from build123d import *

# Parameters (mm, degrees)
SKETCH_1_W      = 8.2
SKETCH_1_H      = 5.2
EXTRUDE_1_DEPTH = 13
SKETCH_2_R      = 2.5
EXTRUDE_2_DEPTH = 6
SKETCH_3_R      = 1.25
EXTRUDE_3_DEPTH = 9.5


with BuildPart() as part:
    # 草圖1 → 填料-伸長1 (new body)
    with BuildSketch(Plane.XY):
        with Locations((-38.465519845, -46.707444045)):
            Rectangle(SKETCH_1_W, SKETCH_1_H)
    extrude(amount=EXTRUDE_1_DEPTH)

    # 草圖2 → 填料-伸長2 (add)
    with BuildSketch(Plane(origin=(0, 0, 0), x_dir=(-1, 0, 0), z_dir=(0, 0, -1))):
        with Locations((38.465519845, -46.707444045)):
            Circle(SKETCH_2_R)
    extrude(amount=EXTRUDE_2_DEPTH)

    # 草圖3 → 填料-伸長3 (add)
    with BuildSketch(Plane(origin=(0, 0, -6), x_dir=(-1, 0, 0), z_dir=(0, 0, -1))):
        with Locations((38.465519845, -46.707444045)):
            Circle(SKETCH_3_R)
    extrude(amount=EXTRUDE_3_DEPTH)


solid = part.part
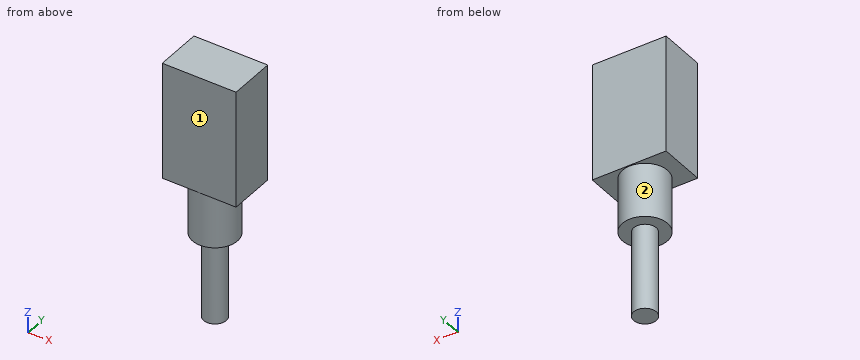
The listing builds one solid part. Answer for the finished solid, in the listing's coordinates (mm). Face numbers are marked on the shaded views. A direction names the side the tool comes from. Round coordinates to 2 decimals unless told otherwise and drop trailing zeros. Order: outer loops, then holes, each group sorted by start corner. A loop starts at its lowest first (then second) coordinate and runs counter-clockwise, first axis right, second up. Notation, with made-up numbers: M -37.5,-5.75 L -16.5,-5.75 A30 ccw -16.5,20.25 Z; hole C 32.5,72.5 d2. An arc over 180 degrees is marked long. Answer in a Markdown table with one row per item. Add a question column.
1) The part is cut by section D-D on x = -39.25. Determine the outline of the cut face in (y, z).
2) The part is cut by section C-C on y = -48.55. Determine the outline of the cut face in (x, z), plus the area to 3 significant figures.
3) Consider line 1 along Z through (x, y) = (-35.5, -48.9); line 2 along Z through (x, y) = (-38.5, -44.8); line 3 along Y through (x, z) = (-40, -3.5). Determine where each line is inside the solid, lowest interval first. Write a range as from..to.
4) Which of the six approach directions +Z, -Z, +X, -X, +Y, -Y give full straight-line access (tool end or side, diameter ignored) to the marked faces 1 and 2?
5) The part is cut by section B-B on y = -45.2. Determine the outline of the cut face in (x, z).
6) The part is cut by section A-A on x = -37.75. Determine the outline of the cut face in (y, z).
Findings below:
| question | item | result |
|---|---|---|
| 1 | outline | M -49.31,0 L -49.08,0 L -49.08,-6 L -47.68,-6 L -47.68,-15.5 L -45.73,-15.5 L -45.73,-6 L -44.33,-6 L -44.33,0 L -44.11,0 L -44.11,13 L -49.31,13 Z |
| 2 | outline | M -42.57,0 L -40.16,0 L -40.16,-6 L -36.78,-6 L -36.78,0 L -34.37,0 L -34.37,13 L -42.57,13 Z |
| 2 | area | 127 mm² |
| 3 | line 1 | z = 0..13 |
| 3 | line 2 | z = -6..13 |
| 3 | line 3 | y = -48.68..-44.73 |
| 4 | face 1 | +Z, -Z, +X, -X, -Y |
| 4 | face 2 | -Z |
| 5 | outline | M -42.57,0 L -40.46,0 L -40.46,-6 L -36.47,-6 L -36.47,0 L -34.37,0 L -34.37,13 L -42.57,13 Z |
| 6 | outline | M -49.31,0 L -49.1,0 L -49.1,-6 L -47.73,-6 L -47.73,-15.5 L -45.68,-15.5 L -45.68,-6 L -44.31,-6 L -44.31,0 L -44.11,0 L -44.11,13 L -49.31,13 Z |
